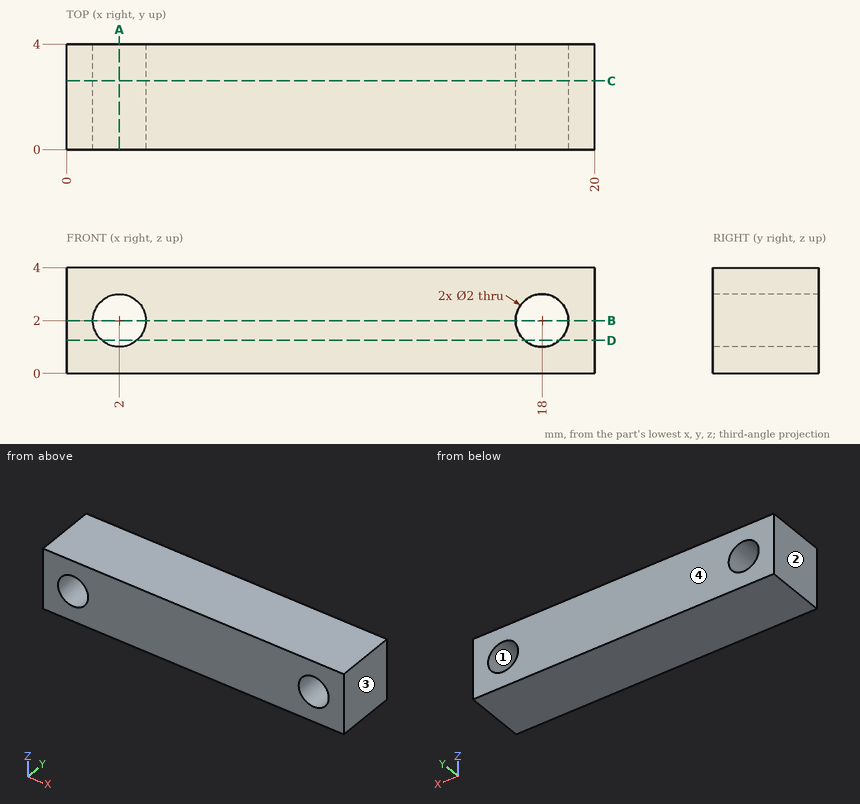
Input: dimensioned drawing with shaded views. Units: mm. Origin: part minimum x, y, z. Give positions to 0.01 mm unless a question says otherwise; leave off trailing zeros. Write each loop counter-clockwise with the first axis right and the second up, starting at its lowest first coordinate (ties: lowest second). Pieces come first, ordered by that corner, then holes. Notation, with made-up numbers: (13.25, 68) -> (70.25, 68) arc R29 cw to (70.25, 106) -> close; hole circle Ø9 at (24.5, -32). An arc over 180 degrees is marked (long way). Return JSON: item names as keys, results as strings. Group by question number.
1. Section D-D, the plane z = 1.25. Output: boundary loops of the cut face in (x, y), then the cut area to 3 significant figures.
2. Section B-B, the plane z = 2. Output: boundary loops of the cut face in (x, y).
3. Mould query, pull axis X, two halves, no side actions, for the marked faces 1, 2, 3 and 4. Classes: +X half, -X half, draft (parallel to the pull), parting line (faces both ways), or undercut.
4. Section C-C, the plane y = 2.6. Output: boundary loops of the cut face in (x, z).
5. Section A-A, the plane x = 2. Output: boundary loops of the cut face in (y, z).
6. Material intervals for line 1 (Z direction, x = 18, y = 0.95); line 2 (X direction, y = 1.75, z = 1.9); line 3 (X direction, y = 2, z = 1.2), sorted ascending. Write a range as from..to.
Determined:
{
 "1": {"outline": "(0, 0) -> (1.34, 0) -> (1.34, 4) -> (0, 4) -> close; (2.66, 0) -> (17.34, 0) -> (17.34, 4) -> (2.66, 4) -> close; (18.66, 0) -> (20, 0) -> (20, 4) -> (18.66, 4) -> close", "area": "69.4 mm2"},
 "2": {"outline": "(0, 0) -> (1, 0) -> (1, 4) -> (0, 4) -> close; (3, 0) -> (17, 0) -> (17, 4) -> (3, 4) -> close; (19, 0) -> (20, 0) -> (20, 4) -> (19, 4) -> close"},
 "3": {"face 1": "undercut", "face 2": "-X half", "face 3": "+X half", "face 4": "draft"},
 "4": {"outline": "(0, 0) -> (20, 0) -> (20, 4) -> (0, 4) -> close; hole circle Ø2 at (2, 2); hole circle Ø2 at (18, 2)"},
 "5": {"outline": "(0, 0) -> (4, 0) -> (4, 1) -> (0, 1) -> close; (0, 3) -> (4, 3) -> (4, 4) -> (0, 4) -> close"},
 "6": {"line 1": "z = 0..1, 3..4", "line 2": "x = 0..1.01, 2.99..17.01, 18.99..20", "line 3": "x = 0..1.4, 2.6..17.4, 18.6..20"}
}
